Job drawing, mm, ordinate dimensions from the low corner. One solid piece. Give positions to 0.01 mm unless a question says otherwise; leave off trailing zeros. Loops run counter-clockwise (first coordinate to the right, second up) from the corner with the lowest first, then second, coordinate; pieces in that order, holes last. Notation, with made-up numbers: M -29,71.5 L -3,71.5 A14 ccw -3,75.5 Z; hole C -26,53.25 d8. An arc over 180 degrees is marked long. One line per question, with ' | ' between items.
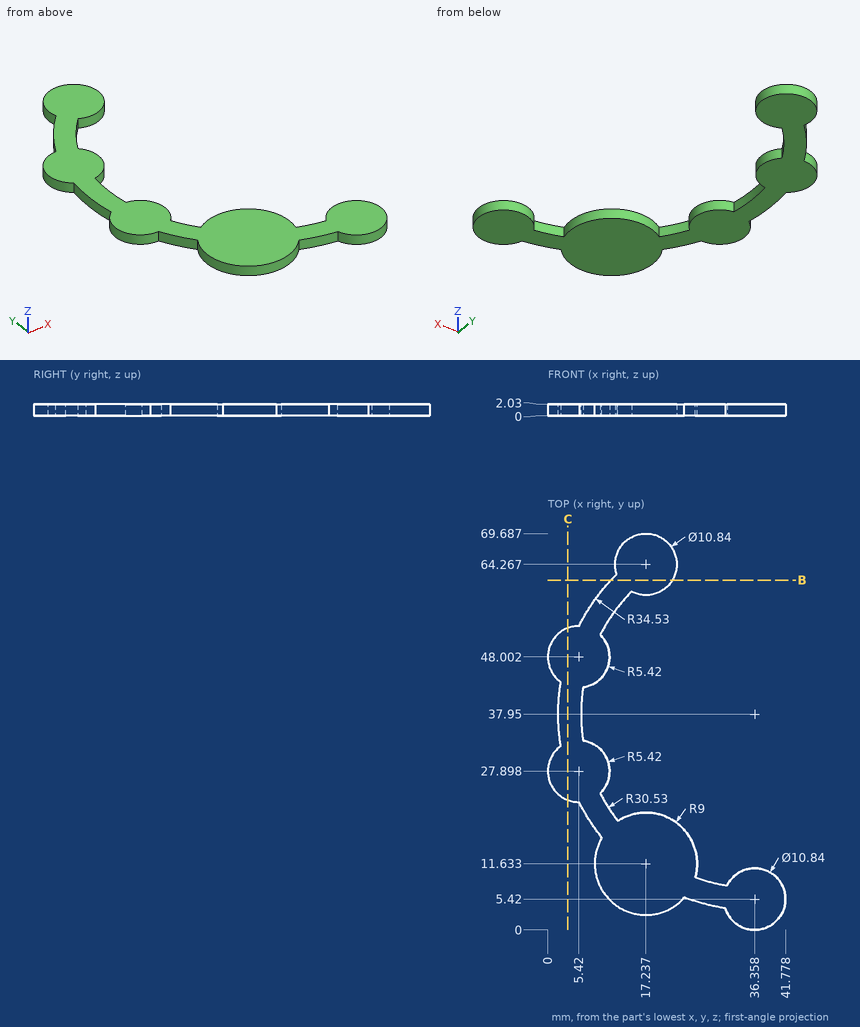
Item 1: Saw through at C-C on x = 3.5. Give the cut face in (y, z).
Conclusion:
outline: M 22.83,0 L 53.07,0 L 53.07,2.03 L 22.83,2.03 Z
Item 2: Drop flat-ended pins along their axis: P1, Ø1, axis at x = 8.5, y = 61, coming from the -Z side; P2, Ø1, axis at x = 6.5, z = 1.5, coming from the -Y side. Give the stop position or say it passes through.
Conclusion:
P1: through | P2: y = 19.77
Item 3: Saw through at B-B on y = 61.5. Give the cut face in (x, z) (1 decimal).
Conclusion:
outline: M 11.1,0 L 21.9,0 L 21.9,2 L 11.1,2 Z
Item 4: Drill centre lines: line 1 along Y through (x, z) = (7, 1.85) (1 decimal); line 2 along Y through (x, z) = (19.5, 1.05); line 3 along X through (y, z) = (9.5, 1) (1 decimal). Where is each one in solid material? Low to high. Write a range as [from, to].
Conclusion:
line 1: [19.8, 33.1], [42.8, 56.1] | line 2: [2.92, 20.34], [59.34, 69.19] | line 3: [8.5, 26], [32.8, 39.9]
